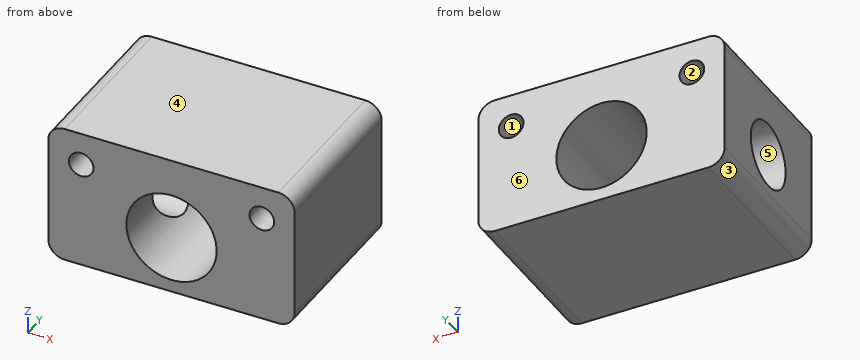
```python
from build123d import *

# Parameters (mm, degrees)
SKETCH_1_W               = 30
SKETCH_1_H               = 17
SKETCH_1_R               = 1.5
SKETCH_1_R_2             = 5.5
EXTRUDE_1_DEPTH          = 20
CUT_EXTRUDE_1_REACH      = 39.044
CUT_EXTRUDE_1_END_RADIUS = 5.5
SKETCH_2_R               = 4
FILLET_1_R               = 2


with BuildPart() as part:
    # 草图1 → 凸台-拉伸1 (new body)
    with BuildSketch(Plane(origin=(0, 0, 0), x_dir=(1, 0, 0), z_dir=(0, 1, 0))):
        Rectangle(SKETCH_1_W, SKETCH_1_H)
        with Locations(Location((-11, -4.5, 0), (0, 0, 270))):
            Circle(SKETCH_1_R, mode=Mode.SUBTRACT)
        with Locations(Location((11, -4.5, 0), (0, 0, 90))):
            Circle(SKETCH_1_R, mode=Mode.SUBTRACT)
        with Locations(Location((0, 1.5, 0), (0, 0, 270))):
            Circle(SKETCH_1_R_2, mode=Mode.SUBTRACT)
    extrude(amount=EXTRUDE_1_DEPTH)

    # 切除-拉伸1: up to this cylinder (the profile starts outside it)
    cut_extrude_1_end = Plane(origin=(0, 10, -1.5), z_dir=(0, -1, 0)) * Cylinder(CUT_EXTRUDE_1_END_RADIUS, 90.088, mode=Mode.PRIVATE)
    # 草图2 → 切除-拉伸1 (cut, up to the surface)
    with BuildSketch(Plane.ZY.offset(15), mode=Mode.PRIVATE) as cut_extrude_1_sk1:
        with Locations((-1.5, 10)):
            Circle(SKETCH_2_R)
    cut_extrude_1_tool1 = extrude(cut_extrude_1_sk1.sketch, amount=-CUT_EXTRUDE_1_REACH, mode=Mode.PRIVATE) - cut_extrude_1_end
    add(cut_extrude_1_tool1.solids().sort_by_distance((-15, 10, -1.5))[0], mode=Mode.SUBTRACT)

    # 圆角1
    fillet_1_edges = [part.edges().sort_by_distance(p)[0] for p in [
        (15, 10, 8.5),
        (-15, 10, 8.5),
        (-15, 10, -8.5),
        (15, 10, -8.5),
    ]]
    fillet(fillet_1_edges, radius=FILLET_1_R)


solid = part.part
```
The listing builds one solid part. Answer for the finished solid, in the listing's coordinates (mm). Face numbers are marked on the shaded views. A direction names the side the tool comes from. Coordinates: 2 decimals unless noted, no trailing zeros. Loops run counter-clockwise (first coordinate to the right, second up) from the corner with the lowest first, then second, coordinate; pieces in that order, holes last. Notation, with made-up numbers: M -16,43.25 L 16,43.25 A19 cw 16,63.25 Z; hole C 25.25,70.5 d7. An arc over 180 degrees is marked long. Answer as a JSON object with one key per item and string values. Group by question number.
Item 1: Determine the mould class of the marked faces 1, 2, 3 and 4 for opening direction Z: +Z half, -Z half, draft (parallel to the pull), parting line (faces both ways), or undercut.
Item 2: Section B-B (y = 10) is taken. Write down the section's boundary in (x, z), and give its area (3 significant figures).
Item 3: Which of the six approach directions +Z, -Z, +X, -X, +Y, -Y give full straight-line access (tool end or side, diameter ignored) to the marked faces 5 and 6?
Item 4: Section A-A (x = -11) is taken. Write down the section's boundary in (y, z).
Item 5: Section C-C (z = -1.5) is taken. Write down the section's boundary in (x, y).
Item 6: Consider L1, parallel to X at y = 13.25, z = 4.5; L2, parallel to X at y = 10.5, z = 5; L3, parallel to Z at x = 11, y = 12.5. Determine where each line is inside the solid, lowest interval first.
Item 7: Section D-D (x = 0) is taken. Write down the section's boundary in (y, z), and give its area (3 significant figures).
Solved:
{
 "1": {"face 1": "undercut", "face 2": "undercut", "face 3": "-Z half", "face 4": "+Z half"},
 "2": {"outline": "M -15,-6.5 A2 ccw -13,-8.5 L 13,-8.5 A2 ccw 15,-6.5 L 15,6.5 A2 ccw 13,8.5 L -13,8.5 A2 ccw -15,6.5 L -15,2.5 L -3.77,2.5 A5.5 cw long -3.77,-5.5 L -15,-5.5 Z; hole C -11,4.5 d3; hole C 11,4.5 d3", "area": "317 mm2"},
 "3": {"face 5": "-X", "face 6": "+Z, -Z, +X, -X, +Y"},
 "4": {"outline": "M 0,-8.5 L 20,-8.5 L 20,3 L 0,3 Z; M 0,6 L 20,6 L 20,8.5 L 0,8.5 Z; hole C 10,-1.5 d8"},
 "5": {"outline": "M -15,0 L -5.5,0 L -5.5,6 L -15,6 Z; M -15,14 L -5.5,14 L -5.5,20 L -15,20 Z; M 5.5,0 L 15,0 L 15,20 L 5.5,20 Z"},
 "6": {"L1": "x = -15 to -12.5, -9.5 to 9.5, 12.5 to 15", "L2": "x = -15 to -12.41, -9.59 to 9.59, 12.41 to 15", "L3": "z = -8.5 to 3, 6 to 8.5"},
 "7": {"outline": "M 0,-8.5 L 20,-8.5 L 20,-7 L 0,-7 Z; M 0,4 L 20,4 L 20,8.5 L 0,8.5 Z", "area": "120 mm2"}
}
